from build123d import *

# Parameters (mm, degrees)
SKETCH1_W           = 22
SKETCH1_H           = 25
SKETCH1_R           = 3.5625
BOSS_EXTRUDE1_DEPTH = 3
CUT_EXTRUDE1_DEPTH  = 2
SKETCH2_W           = 22
SKETCH2_H           = 25
SKETCH2_W_2         = 18
SKETCH2_H_2         = 21
BOSS_EXTRUDE2_DEPTH = 10
FILLET1_R           = 1.5
CHAMFER2_SIZE       = 0.5
FILLET2_R           = 0.5
SKETCH6_W           = 17.056767778
SKETCH6_H           = 17.056767778
CUT_EXTRUDE4_DEPTH  = 3


with BuildPart() as part:
    # Sketch1 → Boss-Extrude1 (new body)
    with BuildSketch(Plane(origin=(0, 0, 0), x_dir=(1, 0, 0), z_dir=(0, 1, 0))):
        with Locations((0, 1.5)):
            Rectangle(SKETCH1_W, SKETCH1_H)
        with Locations(Location((0, 0, 0), (0, 0, 270))):
            Circle(SKETCH1_R, mode=Mode.SUBTRACT)
    extrude(amount=BOSS_EXTRUDE1_DEPTH)

    # 3DSketch1 → Cut-Extrude1 (cut)
    with BuildSketch(Plane(origin=(8.5, 0, -1.375), x_dir=(-0.5881716976750463, 0, 0.8087360843031886), z_dir=(0, -1, 0))):
        Polygon((0, 0), (1.176343395, 1.617472169), (3.400367627, 0), (2.224024232, -1.617472169), align=None)
    extrude(amount=-CUT_EXTRUDE1_DEPTH, mode=Mode.SUBTRACT)

    # Sketch2 → Boss-Extrude2 (add)
    with BuildSketch(Plane.XZ):
        with Locations((0, -1.5)):
            Rectangle(SKETCH2_W, SKETCH2_H)
        with Locations((0, -1.5)):
            Rectangle(SKETCH2_W_2, SKETCH2_H_2, mode=Mode.SUBTRACT)
    extrude(amount=BOSS_EXTRUDE2_DEPTH)

    # Fillet1
    fillet1_edges = [part.edges().sort_by_distance(p)[0] for p in [
        (11, 3, -1.5),
        (0, 3, -14),
        (-11, 3, -1.5),
        (0, 3, 11),
        (-11, -3.5, -14),
        (11, -3.5, -14),
        (11, -3.5, 11),
        (-11, -3.5, 11),
    ]]
    fillet(fillet1_edges, radius=FILLET1_R)

    # Chamfer2
    chamfer2_edges = [part.edges().sort_by_distance(p)[0] for p in [
        (0, 0, -3.5625),
    ]]
    chamfer(chamfer2_edges, length=CHAMFER2_SIZE)

    # Fillet2
    fillet2_edges = [part.edges().sort_by_distance(p)[0] for p in [
        (8.5, 1, -1.375),
        (8.5, 1, 1.375),
        (6.5, 1, 1.375),
        (6.5, 1, -1.375),
    ]]
    fillet(fillet2_edges, radius=FILLET2_R)

    # Sketch6 → Cut-Extrude4 (cut)
    with BuildSketch(Plane(origin=(0, 0, -14), x_dir=(-1, 0, 0), z_dir=(0, 0, -1))):
        with Locations((0, -10)):
            Rectangle(SKETCH6_W, SKETCH6_H)
    extrude(amount=-CUT_EXTRUDE4_DEPTH, mode=Mode.SUBTRACT)


solid = part.part
Model file for the job. Use its own axes, mm. A direction names the side the tool comes from. Round coordinates to 2 decimals unless told otherwise and drop trailing zeros. Loops run counter-clockwise (first coordinate to the right, second up) from the corner with the lowest first, then second, coordinate; pieces in that order, holes last. Notation, with made-up numbers: (61.5, 26) -> (88.5, 26) arc R19 cw to (88.5, 62) -> close; hole circle Ø6 at (5, 16). An arc over 180 degrees is marked (long way). Answer as CSV lines item,"result". Start each with the question number.
1) Mould opens along Z. For faces 1 (the face through (0, -1, -12)), 2 (the face through (0, -1, -14)), 3 (the face through (-11, -4, -2)) say: +Z half, -Z half, draft (parallel to the pull), parting line (faces both ways), or undercut.
2) Slice it at A-A (x = 0). List the corners of the cut face in (y, z), plus the area to 3 significant figures.
3) Pin check, flat tips, straight feed: P1, Ø0.6, axis at y = -7, z = -13, coming from the -X side; P2, Ø0.6, axis at x = 2.5, z = -13, coming from the -Y side; P3, Ø9, axis at x = 2.5, z = 3, coming from the -Y side. Stop position of each tip, or through.
4) Tool access for faces 4 (the face through (-1, -10, 10)), 5 (the face through (7, 2, 0)), 6 (the face through (-8.528, -6, -13)): list every direction of +Z, -Z, +X, -X, +Y, -Y with a clear straight run to the whole face (end or side of a thin tool).
5) Slice it at C-C (z = 0). List the corners of the cut face in (x, y), plus the area to 3 significant figures.
6) Slice it at B-B (y = -0.5). List the corners of the cut face in (x, z).
7) Slice it at D-D (z = 7.5). List the corners of the cut face in (x, y).
8) Probe line 1 along X through (y, z) = (1.45, 0); line 2 along X through (y, z) = (-2.5, -3); line 3 along Y through (x, z) = (6, 6). List the from-to ranges inside material, lowest first.
Filled in:
1,face 1,"undercut"
1,face 2,"-Z half"
1,face 3,"draft"
2,outline,"(-10, 9) -> (0, 9) -> (0, 4.06) -> (0.5, 3.56) -> (3, 3.56) -> (3, 9.5) arc R1.5 ccw to (1.5, 11) -> (-10, 11) -> close; (-1.47, -14) -> (1.5, -14) arc R1.5 ccw to (3, -12.5) -> (3, -3.56) -> (0.5, -3.56) -> (0, -4.06) -> (0, -12) -> (-1.47, -12) -> close"
2,area,"75.4 mm2"
3,P1,"stops at x = -10.99"
3,P2,"stops at y = -1.47"
3,P3,"stops at y = 0"
4,face 4,"+Z, -Z, +X, -X, -Y"
4,face 5,"-Y"
4,face 6,"-Z, -Y"
5,outline,"(-11, -10) -> (-9, -10) -> (-9, 0) -> (-4.06, 0) -> (-3.56, 0.5) -> (-3.56, 3) -> (-9.5, 3) arc R1.5 ccw to (-11, 1.5) -> close; (3.56, 0.5) -> (4.06, 0) -> (6.5, 0) -> (6.5, 2) -> (8.5, 2) -> (8.5, 0) -> (9, 0) -> (9, -10) -> (11, -10) -> (11, 1.5) arc R1.5 ccw to (9.5, 3) -> (3.56, 3) -> close"
5,area,"79.4 mm2"
6,outline,"(-11, -12.5) arc R1.5 ccw to (-9.5, -14) -> (9.5, -14) arc R1.5 ccw to (11, -12.5) -> (11, 9.5) arc R1.5 ccw to (9.5, 11) -> (-9.5, 11) arc R1.5 ccw to (-11, 9.5) -> close; hole (-9, -12) -> (9, -12) -> (9, 9) -> (-9, 9) -> close"
7,outline,"(-11, -10) -> (-9, -10) -> (-9, 0) -> (9, 0) -> (9, -10) -> (11, -10) -> (11, 1.5) arc R1.5 ccw to (9.5, 3) -> (-9.5, 3) arc R1.5 ccw to (-11, 1.5) -> close"
8,line 1,"x = -11 to -3.56, 3.56 to 6.5, 8.5 to 11"
8,line 2,"x = -11 to -9, 9 to 11"
8,line 3,"y = 0 to 3"
